The figure shows three views and two pictorial views of one solid part (mm, origin at its lowest corner). Answer the questions. A direction names the side the tool comes from. Round coordinates to 2 decimals unless told otherwise and drop trailing zeros. Write each loop counter-clockwise with the first axis right and the second up, starting at its lowest first coordinate (ties: lowest second). Pieces come first, ordered by that corner, then holes. Notation, with made-up numbers: (45.5, -5.75) -> (100.5, -5.75) arc R15 cw to (100.5, 18.25) -> close; hole circle Ø3 at (-25, 15.25). An arc over 180 degrees is marked (long way). One line per item, written item: value.
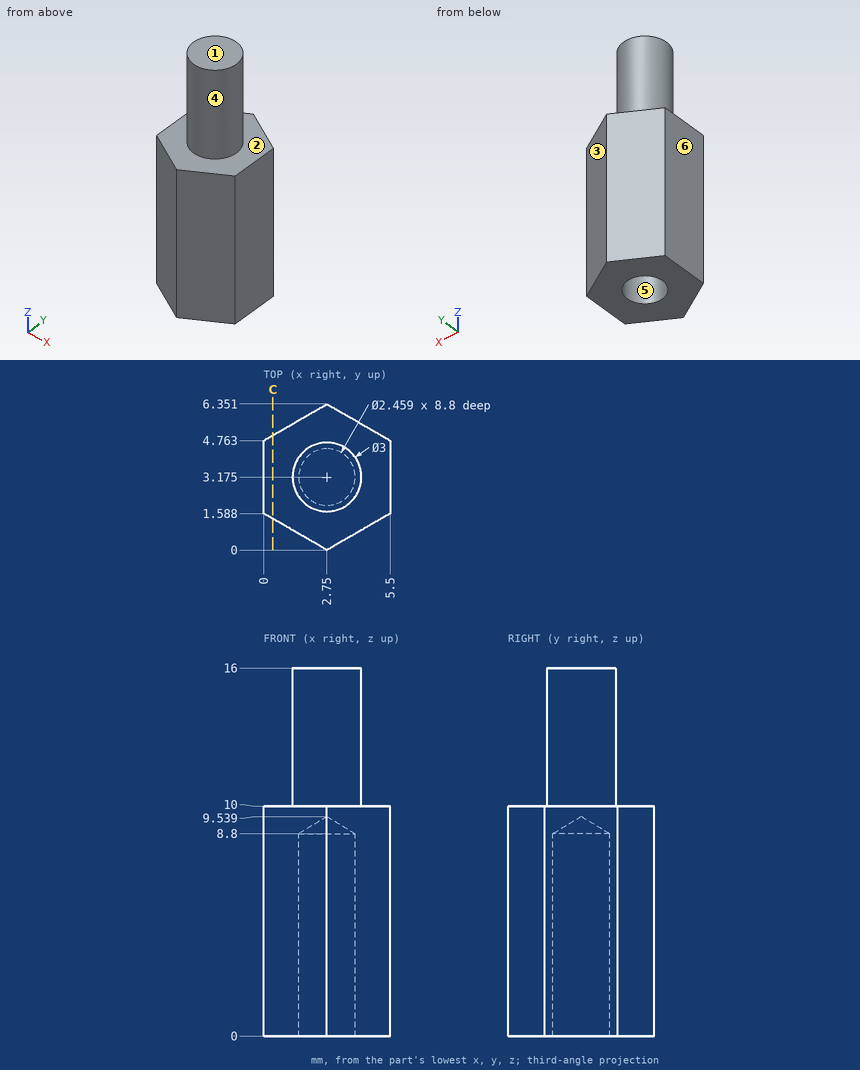
(1) Find section C-C on x = 0.4. Give the vertices of the cut face in (y, z), plus the area to 3 significant figures.
Reported:
outline: (1.36, 0) -> (4.99, 0) -> (4.99, 10) -> (1.36, 10) -> close
area: 36.4 mm2
(2) Flat-ended cylindrical pins translate along their axes: pin 1 Ø1.5 at (x, z) = (1, 3) entering from -Y; pin 2 Ø2 at (x, y) = (2.75, 3.18) entering from -Z (1 decimal). Find the tip coordinate at first contact, or state that the pin passes through.
Reported:
pin 1: stops at y = 0.58
pin 2: stops at z = 8.9
(3) Consider probe 1 along Z at (x, y) = (3.9, 1.75); probe 2 along X at (y, z) = (2.5, 8); probe 3 along X at (y, z) = (4, 6.25). Determine where each line is inside the solid, lowest interval first.
Reported:
probe 1: z = 0 to 10
probe 2: x = 0 to 1.72, 3.78 to 5.5
probe 3: x = 0 to 1.84, 3.66 to 5.5
(4) A tool of negligible diameter and unlimited length cuts with its end or side. For the marked faces 1 and 2, from which of +Z, -Z, +X, -X, +Y, -Y can it reach the whole face along a straight path? Write none if from no direction.
Reported:
face 1: +Z, +X, -X, +Y, -Y
face 2: +Z
(5) For a pull along Y with two mould halves and no side action, classify the marked faces 3, 4, 5 and 6 as pulls with the +Y half, pulls with the -Y half, needs draft (parallel to the pull), parting line crosses it, or undercut.
Reported:
face 3: pulls with the +Y half
face 4: parting line crosses it
face 5: undercut
face 6: needs draft
